Geometry check sheet. Reference: the model listing, model coordinates, mm. Round coordinates to 2 decimals unless told otherwise and drop trailing zeros. Order: outer loops, then holes, each group sorted by start corner. A loop starts at its lowest first (then second) coordinate and runs counter-clockwise, first axis right, second up.
(1) Thickness scan on L1, parallel to Y at x = 9.5, z = 28.5; L2, parallel to Y at x = 21, z = 2; L3, parallel to Z at x = 3.25, y = -12. Record the ranges inside material, lowest first.
(2) Cross-section at B-B on y = -23. Enter the section's corners in (x, z).
(3) Gauge pin test, flat ends, axial feed: P1, Ø6, axis at x = 7.5, z = 26, coming from the -Y side; P2, Ø6, axis at x = 5, z = 17.5, coming from the -Y side; P3, Ø2, axis at x = 8.5, y = -18, coming from the +Z side. Record the tip position at first contact, or that the pin passes through.
(4) Cross-section at A-A on z = 20. Enter the section's corners in (x, y).
from build123d import *

# Parameters (mm, degrees)
F1_DEPTH = 31.75
F4_DEPTH = 25.4


with BuildPart() as f1:
    # F0 (on Top) → F1 (new body)
    with BuildSketch(Plane.XY):
        Polygon((-6.35, 0), (0, 0), (0, 38.1), (-25.4, 38.1), (-25.4, 25.4), (-6.35, 25.4), align=None)
    extrude(amount=F1_DEPTH)


with BuildPart() as f4:
    # F3 (on Right) → F4 (new body)
    with BuildSketch(Plane.YZ):
        Polygon((-25.4, 0), (0, 0), (0, 31.75), (-6.35, 31.75), align=None)
    extrude(amount=F4_DEPTH)


solid = f4.part
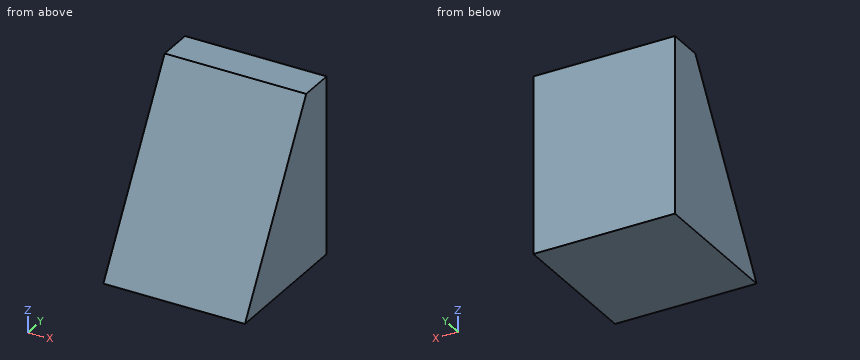
Found:
1. L1: y = -8.3 to 0
1. L2: y = -24.2 to 0
1. L3: z = 0 to 22.33
2. outline: (0, 0) - (25.4, 0) - (25.4, 4) - (0, 4) - close
3. P1: stops at y = -11.6
3. P2: stops at y = -16.7
3. P3: stops at z = 14
4. outline: (0, -13.4) - (25.4, -13.4) - (25.4, 0) - (0, 0) - close
